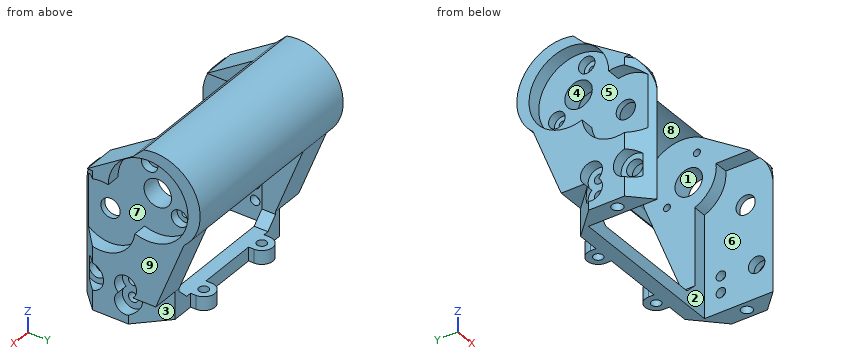
from build123d import *

# Parameters (mm, degrees)
BOSS_EXTRUDE1_DEPTH      = 50
CHAMFER1_SIZE            = 7
SKETCH2_R                = 3.5
CUT_EXTRUDE1_DEPTH       = 66.574385243
SKETCH3_R                = 1.75
CUT_EXTRUDE2_DEPTH       = 66.574385243
SKETCH5_R                = 12.5
CUT_EXTRUDE4_DEPTH       = 5
BOSS_EXTRUDE2_DEPTH      = 12
SKETCH4_W                = 50
SKETCH4_H                = 45
CUT_EXTRUDE3_DEPTH       = 78.43749616
SKETCH7_R                = 1.25
SKETCH7_R_2              = 5
CUT_EXTRUDE5_DEPTH       = 107.904819428
SKETCH8_R                = 14.5
CUT_EXTRUDE6_DEPTH       = 5
SKETCH9_R                = 3
CUT_EXTRUDE7_DEPTH       = 3
SKETCH11_R               = 2
CUT_EXTRUDE8_DEPTH       = 10
BOSS_EXTRUDE3_DEPTH      = 37
SKETCH12_R               = 3
CUT_EXTRUDE9_DEPTH       = 109.932742328
SKETCH13_R               = 5
CUT_EXTRUDE10_DEPTH      = 4
BOSS_EXTRUDE4_DEPTH      = 5
SKETCH16_R               = 1.75
CUT_EXTRUDE12_DEPTH      = 8
CHAMFER2_SIZE            = 4
CUT_EXTRUDE14_DEPTH      = 10
CUT_EXTRUDE15_DEPTH      = 89.087129357
CUT_EXTRUDE15_DEPTH_BACK = 89.087129357


# Read off the part's stored shape, not the designer's step: Mirror1
with BuildPart() as part:
    # Sketch1 → Boss-Extrude1 (new body)
    with BuildSketch(Plane.XY):
        Polygon((-30, 0), (-30, 25), (0, 25), (0, 30), (-37, 30), (-37, 0), align=None)
    extrude(amount=BOSS_EXTRUDE1_DEPTH)

    # Chamfer1
    chamfer1_edges = [part.edges().sort_by_distance(p)[0] for p in [
        (-37, 0, 25),
    ]]
    chamfer(chamfer1_edges, length=CHAMFER1_SIZE - 0.0001)  # a hair under: the kernel refuses the full size

    # Sketch2 → Cut-Extrude1 (cut, through all)
    with BuildSketch(Plane(origin=(-30, 0, 0), x_dir=(0, 0, -1), z_dir=(1, 0, 0))):
        with Locations((-35, 10)):
            Circle(SKETCH2_R)
    extrude(amount=-CUT_EXTRUDE1_DEPTH, mode=Mode.SUBTRACT)

    # Sketch3 → Cut-Extrude2 (cut, through all)
    with BuildSketch(Plane(origin=(-30, 0, 0), x_dir=(0, 0, -1), z_dir=(1, 0, 0))):
        with Locations((-7, 19)):
            Circle(SKETCH3_R)
        with Locations((-13, 19)):
            Circle(SKETCH3_R)
    extrude(amount=-CUT_EXTRUDE2_DEPTH, mode=Mode.SUBTRACT)

    # Sketch5 → Cut-Extrude4 (cut)
    with BuildSketch(Plane.ZY.offset(37)):
        with Locations((35, 10)):
            Circle(SKETCH5_R)
    extrude(amount=-CUT_EXTRUDE4_DEPTH, mode=Mode.SUBTRACT)

    # Sketch6 → Boss-Extrude2 (add)
    with BuildSketch(Plane.ZY.offset(37)):
        with BuildLine():
            Line((43.46072281, 43.154306904), (10, 30))
            Line((10, 30), (36.270468882, 30))
            ThreePointArc((36.270468882, 30), (40.249313761, 20.509847154), (50, 17.220724855))
            Line((50, 17.220724855), (50, 5))
            Line((50, 5), (60.912980238, 21.741514829))
            ThreePointArc((60.912980238, 21.741514829), (60.005508568, 38.820420112), (43.46072281, 43.154306904))
        make_face()
    extrude(amount=-BOSS_EXTRUDE2_DEPTH)

    # Mirror1: part across plane


with BuildPart() as part_1:
    add(part.part)
    add(part.part.mirror(Plane(origin=(0, 0, 0), x_dir=(0, 0, 1), z_dir=(1, 0, 0))))

    # Sketch4 → Cut-Extrude3 (cut, through all)
    with BuildSketch(Plane.XZ.offset(-25)):
        with Locations((0, 27.5)):
            Rectangle(SKETCH4_W, SKETCH4_H)
    extrude(amount=-CUT_EXTRUDE3_DEPTH, mode=Mode.SUBTRACT)

    # Sketch7 → Cut-Extrude5 (cut, through all)
    with BuildSketch(Plane.ZY.offset(37)):
        with Locations(Location((40.983890052, 35.108625208, 0), (0, 0, 270))):
            Circle(SKETCH7_R)
        with Locations(Location((56.547778893, 24.210672918, 0), (0, 0, 270))):
            Circle(SKETCH7_R)
        with Locations(Location((47.045105163, 27.20219293, 0), (0, 0, 270))):
            Circle(SKETCH7_R_2)
    extrude(amount=-CUT_EXTRUDE5_DEPTH, mode=Mode.SUBTRACT)

    # Sketch8 → Cut-Extrude6 (cut)
    with BuildSketch(Plane.ZY.offset(37)):
        with Locations((47.045105163, 27.20219293)):
            Circle(SKETCH8_R)
    cut_extrude6 = extrude(amount=-CUT_EXTRUDE6_DEPTH, mode=Mode.SUBTRACT)

    # Sketch9 → Cut-Extrude7 (cut)
    with BuildSketch(Plane.ZY.offset(32)):
        with Locations(Location((40.983890052, 35.108625208, 0), (0, 0, 270))):
            Circle(SKETCH9_R)
        with Locations(Location((56.547778893, 24.210672918, 0), (0, 0, 270))):
            Circle(SKETCH9_R)
    cut_extrude7 = extrude(amount=-CUT_EXTRUDE7_DEPTH, mode=Mode.SUBTRACT)

    # Sketch11 → Cut-Extrude8 (cut)
    with BuildSketch(Plane(origin=(0, 0, 0), x_dir=(-1, 0, 0), z_dir=(0, 0, -1))):
        with Locations((-33.5, 12)):
            Circle(SKETCH11_R)
    cut_extrude8 = extrude(amount=-CUT_EXTRUDE8_DEPTH, mode=Mode.SUBTRACT)

    # Mirror2: Cut-Extrude6, Cut-Extrude7, Cut-Extrude8 across plane
    add(cut_extrude6.mirror(Plane(origin=(0, 0, 0), x_dir=(0, 0, 1), z_dir=(1, 0, 0))), mode=Mode.SUBTRACT)
    add(cut_extrude7.mirror(Plane(origin=(0, 0, 0), x_dir=(0, 0, 1), z_dir=(1, 0, 0))), mode=Mode.SUBTRACT)
    add(cut_extrude8.mirror(Plane(origin=(0, 0, 0), x_dir=(0, 0, 1), z_dir=(1, 0, 0))), mode=Mode.SUBTRACT)

    # Sketch10 → Boss-Extrude3 (add, symmetric)
    with BuildSketch(Plane(origin=(0, 0, 0), x_dir=(0, 0, -1), z_dir=(1, 0, 0))):
        with BuildLine():
            Line((-43.46072281, 43.154306904), (-36.132650941, 40.273445456))
            ThreePointArc((-36.132650941, 40.273445456), (-56.287994506, 44.345257951), (-64.761056584, 25.609603432))
            Line((-64.761056584, 25.609603432), (-60.912980238, 21.741514829))
            ThreePointArc((-60.912980238, 21.741514829), (-60.005508568, 38.820420112), (-43.46072281, 43.154306904))
        make_face()
    extrude(amount=BOSS_EXTRUDE3_DEPTH, both=True)

    # Sketch12 → Cut-Extrude9 (cut, through all)
    with BuildSketch(Plane(origin=(37, 0, 0), x_dir=(0, 0, -1), z_dir=(1, 0, 0))):
        with Locations(Location((-12, 6, 0), (0, 0, 19.471220634))):
            Circle(SKETCH12_R)
    extrude(amount=-CUT_EXTRUDE9_DEPTH, mode=Mode.SUBTRACT)

    # Sketch13 → Cut-Extrude10 (cut)
    with BuildSketch(Plane(origin=(37, 0, 0), x_dir=(0, 0, -1), z_dir=(1, 0, 0))):
        with Locations((-12, 6)):
            Circle(SKETCH13_R)
        with BuildLine():
            ThreePointArc((-10, 21.645751311), (-17, 19), (-10, 16.354248689))
            ThreePointArc((-10, 16.354248689), (-3, 19), (-10, 21.645751311))
        make_face()
    cut_extrude10 = extrude(amount=-CUT_EXTRUDE10_DEPTH, mode=Mode.SUBTRACT)

    # Mirror3: Cut-Extrude10 across plane
    add(cut_extrude10.mirror(Plane(origin=(0, 0, 0), x_dir=(0, 0, 1), z_dir=(1, 0, 0))), mode=Mode.SUBTRACT)

    # Sketch15 → Boss-Extrude4 (add)
    with BuildSketch(Plane(origin=(0, 0, 0), x_dir=(-1, 0, 0), z_dir=(0, 0, -1))):
        with BuildLine():
            Line((-19, 32), (-19, 30))
            Line((-19, 30), (-11, 30))
            Line((-11, 30), (-11, 32))
            ThreePointArc((-11, 32), (-15, 36), (-19, 32))
        make_face()
        with BuildLine():
            Line((11, 30), (11, 32))
            ThreePointArc((11, 32), (15, 36), (19, 32))
            Line((19, 32), (19, 30))
            Line((19, 30), (11, 30))
        make_face()
    extrude(amount=-BOSS_EXTRUDE4_DEPTH)

    # Sketch16 → Cut-Extrude12 (cut)
    with BuildSketch(Plane(origin=(0, 0, 0), x_dir=(-1, 0, 0), z_dir=(0, 0, -1))):
        with Locations((-15, 32)):
            Circle(SKETCH16_R)
        with Locations((15, 32)):
            Circle(SKETCH16_R)
    extrude(amount=-CUT_EXTRUDE12_DEPTH, mode=Mode.SUBTRACT)

    # Chamfer2
    chamfer2_edges = [part_1.edges().sort_by_distance(p)[0] for p in [
        (25, 27.5, 5),
        (-25, 27.5, 5),
    ]]
    chamfer(chamfer2_edges, length=CHAMFER2_SIZE)

    # Sketch17 → Cut-Extrude14 (cut)
    with BuildSketch(Plane(origin=(0, 0, 0), x_dir=(-1, 0, 0), z_dir=(0, 0, -1))):
        Polygon((-37, 20), (-37, 30), (-27, 30), align=None)
        Polygon((37, 30), (27, 30), (37, 20), align=None)
    extrude(amount=-CUT_EXTRUDE14_DEPTH, mode=Mode.SUBTRACT)

    # Sketch18 → Cut-Extrude15 (cut, two sides: drawn at the far end of the back side and taken through both)
    with BuildSketch(Plane(origin=(0, 0, 0), x_dir=(0, 0, -1), z_dir=(1, 0, 0)).offset(-CUT_EXTRUDE15_DEPTH_BACK)):
        with BuildLine():
            Line((-38.575094924, 0), (-50, 0))
            Line((-50, 0), (-53.770765751, 10.784701278))
            ThreePointArc((-53.770765751, 10.784701278), (-47.891990779, 2.970190216), (-38.575094924, 0))
        make_face()
    extrude(amount=CUT_EXTRUDE15_DEPTH + CUT_EXTRUDE15_DEPTH_BACK, mode=Mode.SUBTRACT)


solid = part_1.part
For this review, take the finished solid that the model builds, in its own axes (mm). Face numbers are marked on the shaded views. A direction names the side the tool comes from. Round coordinates to 2 decimals unless told otherwise and drop trailing zeros. Loops run counter-clockwise (first coordinate to the right, second up) from the corner with the lowest first, then second, coordinate; pieces in that order, holes last. Notation, with made-up numbers: (-20, 72.25) - (0, 72.25) arc R7 cw to (0, 83.25) - close; hole circle Ø6 at (44, 62.25). An arc over 180 degrees is marked (long way). Use one line per item in the form item = value.
Item 1: Consider section B-B on x = 24. Write out the cut boundary in (y, z), then the cut area to 3 significant figures.
Answers:
outline = (21.74, 60.91) arc R14.5 cw to (43.15, 43.46) - (40.27, 36.13) arc R16.5 ccw to (25.61, 64.76) - close; (25, 0) - (30, 0) - (30, 8) - (25, 8) - close
area = 123 mm^2
Item 2: Consider section D-D on x = 1. Write out the cut boundary in (y, z).
Answers:
outline = (21.74, 60.91) arc R14.5 cw to (43.15, 43.46) - (40.27, 36.13) arc R16.5 ccw to (25.61, 64.76) - close; (25, 0) - (30, 0) - (30, 5) - (25, 5) - close
Item 3: Consider section A-A on x = -15. Write out the cut boundary in (y, z), then the cut area to 3 significant figures.
Answers:
outline = (21.74, 60.91) arc R14.5 cw to (43.15, 43.46) - (40.27, 36.13) arc R16.5 ccw to (25.61, 64.76) - close; (25, 0) - (30.25, 0) - (30.25, 5) - (25, 5) - close; (33.75, 0) - (36, 0) - (36, 5) - (33.75, 5) - close
area = 120 mm^2
Item 4: Tool access review of the marked faces 5, 6, 7, 8 and 9: name each direction out of +Z, -Z, +X, -X, +Y, -Y from which nothing blocks a thin tool from reaching the whole face with its end or side.
Answers:
face_5 = -X
face_6 = -Z, -Y
face_7 = +X
face_8 = none
face_9 = +Z, -Z, +X, +Y, -Y
Item 5: Mouldability with a two-part tool opening along Y and no side actions: class the marked faces 1, 2, 3 and 4 as +Y half, -Y half, draft (parallel to the pull), parting line (faces both ways), or undercut.
Answers:
face_1 = undercut
face_2 = -Y half
face_3 = +Y half
face_4 = undercut
Item 6: Clearance check with flat-ended pins moving along their axes: P1, Ø6, axis at y = 5.5, z = 44, coming from the +X side; P2, Ø1.6, axis at y = 30.5, z = 1.5, coming from the -X side; P3, Ø9, axis at y = 6, z = 12, coming from the -X side. State where each tip first meets the part, or that it passes through.
Answers:
P1 = 36.22
P2 = -27.3
P3 = -33
Item 7: For line 1 (X direction, y = 2, z = 39); line 2 (Y direction, x = -31.6, z = 12); line 3 (X direction, y = 42.5, z = 42.5), list the stretches that pass through material, from the lowest coordinate up.
Answers:
line_1 = -32 to -30, 30 to 32
line_2 = 1.6 to 3, 9 to 17.56, 20.44 to 30.79
line_3 = -37 to -25, 25 to 37
Item 8: Consider section C-C on z = 45.5. Write out the cut boundary in (x, y).
Answers:
outline = (-37, 41.62) - (-32, 41.62) - (-32, 31.96) - (-25, 31.96) - (-25, 43.79) - (25, 43.79) - (25, 31.96) - (32, 31.96) - (32, 41.62) - (37, 41.62) - (37, 45.83) - (-37, 45.83) - close; (-33.22, 3.22) - (-31.57, 1.57) - (-30, 1.57) - (-30, 17.59) - (-25, 17.59) - (-25, 22.45) - (-32, 22.45) - (-32, 3.22) - close; (25, 17.59) - (30, 17.59) - (30, 1.57) - (31.57, 1.57) - (33.22, 3.22) - (32, 3.22) - (32, 22.45) - (25, 22.45) - close
